Design review of the part built by this model. Coordinates are the model's own, in mm. Face numbers are marked on the shaded views. A direction names the side the tool comes from. Coordinates: 2 decimals unless noted, no trailing zeros. Order: outer loops, then holes, each group sorted by start corner. A loop starts at its lowest first (then second) coordinate and runs counter-clockwise, first axis right, second up. Notation, with made-up numbers: M 28,-10.75 L 70,-10.75 A24 ccw 70,16.25 Z; hole C 57.25,38.25 d1. An arc over 180 degrees is marked long. Use CSV: the item, a comma, the result in double quotes.
```python
from build123d import *

# Parameters (mm, degrees)
F1_DEPTH = 14.5
F2_DEPTH = 14.5
F4_DEPTH = 7
F5_R     = 0.9
F6_DEPTH = 2
F7_SIZE  = 1.5
F8_R     = 1


with BuildPart() as f1:
    # F0 (on Top) → F1 (new body)
    with BuildSketch(Plane.XY):
        with BuildLine():
            Line((5, 4.472136), (5, 15))
            Line((5, 15), (5, 16.972136))
            Line((5, 16.972136), (3, 16.972136))
            Line((3, 16.972136), (3, 15))
            Line((3, 15), (3, 13.645751))
            ThreePointArc((3, 13.645751), (4, 11), (3, 8.354249))
            Line((3, 8.354249), (3, 2.95804))
            Line((3, 2.95804), (5, 2.95804))
            ThreePointArc((5, 2.95804), (7.436492, 2.291288), (8.5, 0))
            ThreePointArc((8.5, 0), (7.436492, -2.291288), (5, -2.95804))
            Line((5, -2.95804), (3, -2.95804))
            Line((3, -2.95804), (3, -8.354249))
            ThreePointArc((3, -8.354249), (4, -11), (3, -13.645751))
            Line((3, -13.645751), (3, -15))
            Line((3, -15), (3, -16.972136))
            Line((3, -16.972136), (5, -16.972136))
            Line((5, -16.972136), (5, -15))
            Line((5, -15), (5, -4.472136))
            ThreePointArc((5, -4.472136), (8.5, -3.354102), (10, 0))
            ThreePointArc((10, 0), (8.5, 3.354102), (5, 4.472136))
        make_face()
    extrude(amount=F1_DEPTH)

    # F0 (on Top) → F2 (join)
    with BuildSketch(Plane.XY):
        with BuildLine():
            ThreePointArc((3, 8.354249), (4, 11), (3, 13.645751))
            ThreePointArc((3, 13.645751), (0.408409, 14.979096), (-2.4, 14.2))
            Line((-2.4, 14.2), (-1.5, 13))
            ThreePointArc((-1.5, 13), (2.5, 11), (-1.5, 9))
            Line((-1.5, 9), (-2.4, 7.8))
            ThreePointArc((-2.4, 7.8), (0.408409, 7.020904), (3, 8.354249))
        make_face()
        with BuildLine():
            ThreePointArc((-2.4, -14.2), (0.408409, -14.979096), (3, -13.645751))
            ThreePointArc((3, -13.645751), (4, -11), (3, -8.354249))
            ThreePointArc((3, -8.354249), (0.408409, -7.020904), (-2.4, -7.8))
            Line((-2.4, -7.8), (-1.5, -9))
            ThreePointArc((-1.5, -9), (2.5, -11), (-1.5, -13))
            Line((-1.5, -13), (-2.4, -14.2))
        make_face()
    extrude(amount=F2_DEPTH)

    # F3 (on face) → F4 (cut)
    with BuildSketch(Plane.XY.offset(14.5)):
        with BuildLine():
            Line((5, -2.95804), (5, -4.472136))
            ThreePointArc((5, -4.472136), (10, 0), (5, 4.472136))
            Line((5, 4.472136), (5, 2.95804))
            ThreePointArc((5, 2.95804), (8.5, 0), (5, -2.95804))
        make_face()
    extrude(amount=-F4_DEPTH, mode=Mode.SUBTRACT)

    # F5 (on face) → F6 (cut)
    with BuildSketch(Plane.YZ.offset(5)):
        with Locations((-14.972136, 7.25)):
            Circle(F5_R)
        with Locations((-6.472136, 7.25)):
            Circle(F5_R)
        with Locations((6.472136, 7.25)):
            Circle(F5_R)
        with Locations((14.972136, 7.25)):
            Circle(F5_R)
    extrude(amount=-F6_DEPTH, mode=Mode.SUBTRACT)

    # F7
    f7_edges = [f1.edges().sort_by_distance(p)[0] for p in [
        (4, -16.972136, 14.5),
        (4, -16.972136, 0),
        (4, 16.972136, 0),
        (4, 16.972136, 14.5),
        (4, 2.95804, 14.5),
        (4, -2.95804, 14.5),
    ]]
    chamfer(f7_edges, length=F7_SIZE)

    # F8
    f8_edges = [f1.edges().sort_by_distance(p)[0] for p in [
        (-1.5, -9, 7.25),
        (-1.5, 13, 7.25),
        (-1.5, -13, 7.25),
        (-1.5, 9, 7.25),
        (5, -3.715088, 7.5),
        (5, 3.715088, 7.5),
        (3, 2.95804, 6.5),
        (3, -2.95804, 6.5),
    ]]
    fillet(f8_edges, radius=F8_R)


solid = f1.part
```
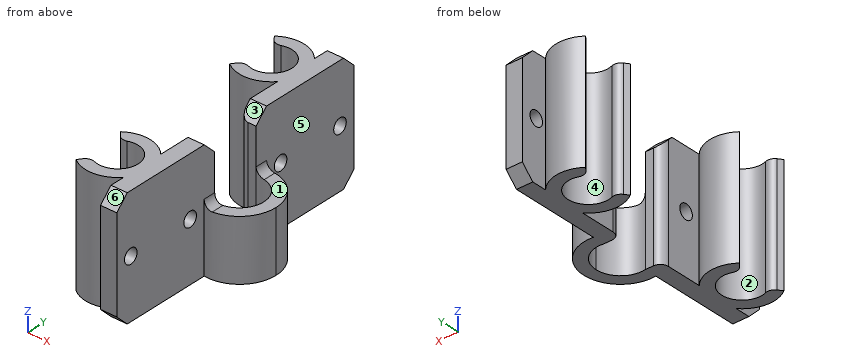
(1) Add section C-C on y = 5. State the section outline as (x, z) points, and give its area (3 significant figures).
The answers:
outline,"M 3,0 L 5,0 L 5,14.5 L 3,14.5 Z"
area,"29.0 mm2"
(2) For the marked faces 1, 2 and 3, list the 3-axis set-ups (+Z, -Z, +X, -X, +Y, -Y) from which the entire face can be reached by the end or side of a thin tool; tool diameter is ignored.
The answers:
face 1,"+Z, +X, +Y, -Y"
face 2,"+Z, -Z"
face 3,"+Z, +X, -X"
(3) Clearance check with flat-ended pins moving along their axes: P1, Ø8, axis at y = -11, z = 3, coming from the +X side; P2, Ø1.5, axis at x = 0, y = -11.5, coming from the +Z side; P3, Ø4, axis at y = -13.5, z = 7.5, coming from the -X side; P4, Ø1.1, axis at y = -14.97, z = 7.25, coming from the +X side. State where each tip first meets the part, or that it passes through.
The answers:
P1,"stops at x = 5"
P2,"passes through"
P3,"stops at x = -2.4"
P4,"stops at x = 2.07"
(4) Add section B-B on z = 12.25. State the section outline as (x, y) points, and give its area (3 significant figures).
The answers:
outline,"M -2.4,-14.2 A4 ccw 3,-13.65 L 3,-16.97 L 5,-16.97 L 5,-2.96 L 4,-2.96 A1 ccw 3,-3.96 L 3,-8.35 A4 ccw -2.4,-7.8 L -2.01,-8.32 A1 ccw -0.87,-8.65 A2.5 cw long -0.87,-13.35 A1 ccw -2.01,-13.68 Z; M -2.4,7.8 A4 ccw 3,8.35 L 3,3.96 A1 ccw 4,2.96 L 5,2.96 L 5,16.97 L 3,16.97 L 3,13.65 A4 ccw -2.4,14.2 L -2.01,13.68 A1 ccw -0.87,13.35 A2.5 cw long -0.87,8.65 A1 ccw -2.01,8.32 Z"
area,"91.0 mm2"
(5) Add section A-A on x = 0. State the section outline as (y, z) points, and give its area (3 significant figures).
The answers:
outline,"M -15,0 L -13.5,0 L -13.5,14.5 L -15,14.5 Z; M -8.5,0 L -7,0 L -7,14.5 L -8.5,14.5 Z; M 7,0 L 8.5,0 L 8.5,14.5 L 7,14.5 Z; M 13.5,0 L 15,0 L 15,14.5 L 13.5,14.5 Z"
area,"87.0 mm2"
(6) The part is to be moulded in two halves that separate along Y. For the marked faces 4, 5 and 6, say which applies: pulls with the +Y half, pulls with the -Y half, needs draft (parallel to the pull), parting line crosses it, or undercut.
The answers:
face 4,"undercut"
face 5,"needs draft"
face 6,"pulls with the -Y half"
(7) Wall thickness on probe 1 along Y at (x, z) = (0, 12.5); probe 2 along Z at (x, y) = (3.5, 6.5); probe 3 along Y at (x, z) = (1.5, 11.75): over which ranges is each line inside the solid? List them lowest first.
The answers:
probe 1,"y = -15 to -13.5, -8.5 to -7, 7 to 8.5, 13.5 to 15"
probe 2,"z = 0 to 6.35, 8.15 to 14.5"
probe 3,"y = -14.71 to -13, -9 to -7.29, 7.29 to 9, 13 to 14.71"
